The listing builds one solid part. Answer for the finished solid, in the listing's coordinates (mm). Face numbers are marked on the shaded views. A direction names the side the tool comes from. Give positions to 0.01 mm unless a question says otherwise; leave off trailing zeros. Write each loop counter-clockwise with the first axis right and the second up, starting at its lowest first coordinate (ties: lowest second). Pieces come first, ordered by that corner, then holes.
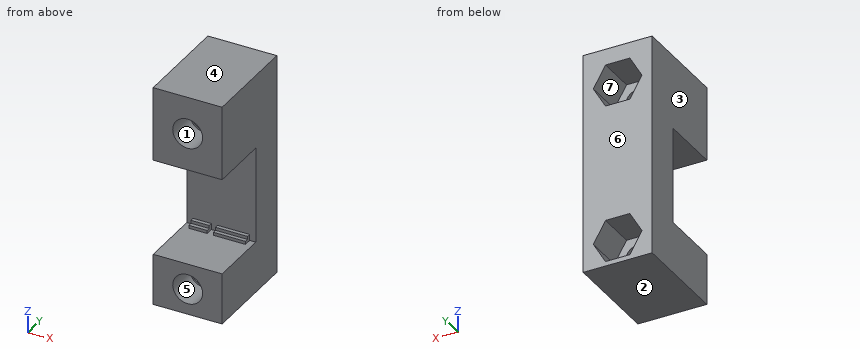
Autodesk Inventor part; units mm, degrees
ref_plane "YZ Plane" through (0, 0, 0) normal (1, 0, 0) x (0, 1, 0)
ref_plane "XZ Plane" through (0, 0, 0) normal (0, 1, 0) x (-1, 0, 0)
ref_plane "XY Plane" through (0, 0, 0) normal (0, 0, 1) x (1, 0, 0)
sketch "Szkic1" plane through (0, 0, 0) normal (1, 0, 0) x (0, 1, 0)
  line L0 (-4, 6.3) -> (4, 6.3)
  line L1 (4, 6.3) -> (4, -6.3)
  line L2 (4, -6.3) -> (-4, -6.3)
  line L3 (-4, 6.3) -> (-4, 13)
  line L4 (-4, -6.3) -> (-4, -13)
  line L5 (-1, -13) -> (-1, -9.3)
  line L6 (-1, -9.3) -> (7, -9.3)
  line L7 (7, -9.3) -> (7, 9.3)
  line L8 (7, 9.3) -> (-1, 9.3)
  line L9 (-1, 9.3) -> (-1, 13)
  line L10 (-4, 13) -> (-1, 13)
  line L11 (-4, -13) -> (-1, -13)
  point P0 (0, 0)
  point P1 (0, 6.3)
  point P2 (4, 0)
  dimension "d0" = 8
  dimension "d1" = 12.6
  dimension "d2" = 6.7
  dimension "d3" = 6.7
  dimension "d4" = 3
extrude "Wyciągnięcie proste1" add sketch "Szkic1" along normal blind 9
sketch "Szkic2" plane through (0, 4, -6.3) normal (0, -1, 0) x (1, 0, 0)
  line L0 (0, 12.6) -> (0, 0)
  line L1 (0, 0) -> (9, 0)
  line L2 (9, 12.6) -> (9, 0)
  line L3 (0, 12.6) -> (9, 12.6)
  line L4 (8.2, 12.6) -> (8.2, 0)
  line L5 (4, 12.6) -> (4, 0)
  line L6 (3.2, 12.6) -> (3.2, 0)
  line L7 (0.8, 0) -> (0.8, 12.6)
  line L8 (0.8, 12.6) -> (3.2, 12.6)
  line L9 (3.2, 12.6) -> (3.2, 11.8)
  line L10 (3.2, 11.8) -> (0.8, 11.8)
  line L11 (0.8, 11.8) -> (0.8, 12.6)
  line L12 (0.8, 0) -> (3.2, 0)
  line L13 (3.2, 0) -> (3.2, 0.8)
  line L14 (3.2, 0.8) -> (0.8, 0.8)
  line L15 (0.8, 0.8) -> (0.8, 0)
  line L16 (4, 12.6) -> (8.2, 12.6)
  line L17 (8.2, 12.6) -> (8.2, 11.8)
  line L18 (8.2, 11.8) -> (4, 11.8)
  line L19 (4, 11.8) -> (4, 12.6)
  line L20 (4, 0) -> (8.2, 0)
  line L21 (8.2, 0) -> (8.2, 0.8)
  line L22 (8.2, 0.8) -> (4, 0.8)
  line L23 (4, 0.8) -> (4, 0)
  point P0 (0, 6.3)
  point P1 (4, 0.8)
  point P2 (0.8, 0.8)
  point P3 (0.8, 11.8)
  dimension "d7" = 0.8
  dimension "d8" = 4.2
  dimension "d9" = 0.8
  dimension "d10" = 2.4
  dimension "d11" = 0.8
  dimension "d12" = 0.8
  dimension "d13" = 0.8
  dimension "d14" = 0.8
extrude "Wyciągnięcie proste2" add sketch "Szkic2" along normal blind 0.5 contours L3 L6 L10 L7 | L7 L14 L6 L1 | L3 L4 L18 L5 | L5 L22 L4 L1
sketch "Szkic3" plane through (0, 3.5, -6.3) normal (0, -1, 0) x (1, 0, 0)
  line L0 (8.2, 11.8) -> (8.2, 12.6)
  line L1 (4, 12.6) -> (8.2, 12.6)
  line L2 (4, 12.6) -> (4, 11.8)
  line L3 (4, 11.8) -> (8.2, 11.8)
  line L4 (3.2, 11.8) -> (3.2, 12.6)
  line L5 (0.8, 12.6) -> (3.2, 12.6)
  line L6 (0.8, 12.6) -> (0.8, 11.8)
  line L7 (0.8, 11.8) -> (3.2, 11.8)
  line L8 (0.8, 0.8) -> (0.8, 0)
  line L9 (3.2, 0) -> (0.8, 0)
  line L10 (3.2, 0) -> (3.2, 0.8)
  line L11 (3.2, 0.8) -> (0.8, 0.8)
  line L12 (4, 0.8) -> (4, 0)
  line L13 (8.2, 0) -> (4, 0)
  line L14 (8.2, 0) -> (8.2, 0.8)
  line L15 (8.2, 0.8) -> (4, 0.8)
  line L16 (8.2, 12.6) -> (8.2, 11.8)
  line L17 (8.2, 12.2) -> (0.8, 12.2)
  line L18 (8.2, 0.4) -> (0.8, 0.4)
  point P0 (0, 6.3)
  point P1 (4, 0.4)
  point P2 (3.2, 0.4)
  point P3 (4, 12.2)
  point P4 (3.2, 12.2)
extrude "Wyciągnięcie proste3" add sketch "Szkic3" along normal blind 0.5 contours L17 L6 L5 L4 | L17 L2 L1 L0 | L18 L14 L13 L12 | L18 L10 L9 L8
sketch "Szkic4" plane through (9, 0, 0) normal (1, 0, 0) x (0, 0, -1)
  line L0 (-6.3, -4) -> (-6.3, 4)
  line L1 (-6.3, 4) -> (6.3, 4)
  line L2 (6.3, 4) -> (6.3, -4)
  line L3 (6.3, -4) -> (13, -4)
  line L4 (13, -4) -> (13, -1)
  line L5 (13, -1) -> (9.3, -1)
  line L6 (9.3, -1) -> (9.3, 7)
  line L7 (9.3, 7) -> (-9.3, 7)
  line L8 (-9.3, 7) -> (-9.3, -1)
  line L9 (-9.3, -1) -> (-13, -1)
  line L10 (-13, -1) -> (-13, -4)
  line L11 (-13, -4) -> (-6.3, -4)
  line L12 (-13, -1) -> (13, -1)
  line L13 (13, -1) -> (13, 9)
  line L14 (13, 9) -> (-13, 9)
  line L15 (-13, 9) -> (-13, -1)
  point P0 (0, 0)
  dimension "d19" = 10
extrude "Wyciągnięcie proste4" add sketch "Szkic4" against normal up to surface (9 mm away) contours L9 L15 L14 L13 L5 L6 L7 L8
sketch "Szkic5" plane through (0, -4, 13) normal (0, 0, 1) x (1, 0, 0)
  line L0 (0, 0) -> (0, 13)
  line L1 (0, 0) -> (9, 0)
  line L2 (9, 13) -> (9, 0)
  line L3 (9, 13) -> (0, 13)
  point P0 (0, 4)
extrude "Wyciągnięcie proste5" add sketch "Szkic5" along normal blind 3
sketch "Szkic6" plane through (0, -4, -13) normal (0, -1, 0) x (1, 0, 0)
  line L0 (0, 0) -> (9, 0)
  line L1 (0, 6.7) -> (9, 6.7)
  line L2 (0, 19.3) -> (9, 19.3)
  line L3 (0, 29) -> (9, 29)
  line L4 (4.5, 0) -> (4.5, 6.7) construction
  line L5 (4.5, 19.3) -> (4.5, 29) construction
  point P0 (0, 13)
  point P1 (4.5, 3.35)
  point P2 (4.5, 24.15)
hole "Otwór1" at (4.5, -4, -9.65) at (4.5, -4, 11.15) direction (0, 1, 0) diameter 3.5 depth 8 counterbore diameter 3.9 counterbore depth 4
sketch "Szkic7" plane through (0, 9, -13) normal (0, 1, 0) x (1, 0, 0)
  circle A0 centre (4.5, -3.35) radius 1.75
  circle A1 centre (4.5, -24.15) radius 1.75
  circle A2 centre (4.5, -3.35) radius 2.75
  circle A3 centre (4.5, -24.15) radius 2.75
  line L0 (6.0877, -0.6) -> (7.6754, -3.35)
  line L1 (7.6754, -3.35) -> (6.0877, -6.1)
  line L2 (6.0877, -6.1) -> (2.9123, -6.1)
  line L3 (2.9123, -6.1) -> (1.3246, -3.35)
  line L4 (1.3246, -3.35) -> (2.9123, -0.6)
  line L5 (2.9123, -0.6) -> (6.0877, -0.6)
  line L6 (2.9123, -26.9) -> (1.3246, -24.15)
  line L7 (1.3246, -24.15) -> (2.9123, -21.4)
  line L8 (2.9123, -21.4) -> (6.0877, -21.4)
  line L9 (6.0877, -21.4) -> (7.6754, -24.15)
  line L10 (7.6754, -24.15) -> (6.0877, -26.9)
  line L11 (6.0877, -26.9) -> (2.9123, -26.9)
  point P0 (0, -13)
  point P1 (4.5, -0.6)
  point P2 (4.5, -26.9)
  dimension "d31" = 5.5
  dimension "d32" = 5.5
extrude "Wyciągnięcie proste6" cut sketch "Szkic7" against normal blind 5 contours A0 | A1 | A2 | A2 L0 L1 | A2 L5 L0 | L1 L2 A2 | A2 L4 L5 | L2 L3 A2 | A2 L3 L4 | A3 | A3 L9 L10 | A3 L8 L9 | L10 L11 A3 | A3 L7 L8 | L11 L6 A3 | A3 L6 L7
properties part number "motor_bracket"
Item 1: A cutting plane is placed at B-B, the plane y = 5. Give the vertices of the cut face in (x, z).
Conclusion:
outline: (0, -13) - (9, -13) - (9, 16) - (0, 16) - close; hole (1.32, -9.65) - (2.91, -12.4) - (6.09, -12.4) - (7.68, -9.65) - (6.09, -6.9) - (2.91, -6.9) - close; hole (1.32, 11.15) - (2.91, 8.4) - (6.09, 8.4) - (7.68, 11.15) - (6.09, 13.9) - (2.91, 13.9) - close
Item 2: Consider probe 1 along Z at (x, y) = (3.75, 4.75); probe 2 along Z at (x, y) = (4.5, -1.8); probe 3 along Z at (x, y) = (4.5, 2.1). Determine where each line is inside the solid, lowest interval first.
Conclusion:
probe 1: z = -13 to -12.4, -6.9 to 8.4, 13.9 to 16
probe 2: z = -13 to -11.6, -7.7 to -6.3, 6.3 to 9.2, 13.1 to 16
probe 3: z = -13 to -11.4, -7.9 to -6.3, 6.3 to 9.4, 12.9 to 16
Item 3: Determine the mould class of the marked faces 1, 2, 3 and 4 for opening direction Z: pulls with the +Z half, pulls with the -Z half, needs draft (parallel to the pull), parting line crosses it, or undercut.
Conclusion:
face 1: undercut
face 2: pulls with the -Z half
face 3: needs draft
face 4: pulls with the +Z half
Item 4: Which of the six approach directions +Z, -Z, +X, -X, +Y, -Y give full straight-line access (tool end or side, diameter ignored) to the marked faces 5, 6 and 7?
Conclusion:
face 5: -Y
face 6: +Z, -Z, +X, -X, +Y
face 7: +Y
Item 5: A cutting plane is placed at A-A, the plane y = -1.5. Give the vertices of the cut face in (x, z), plus the area to 3 significant figures.
Conclusion:
outline: (0, -13) - (9, -13) - (9, -6.3) - (0, -6.3) - close; (0, 6.3) - (9, 6.3) - (9, 16) - (0, 16) - close; hole circle Ø3.9 at (4.5, -9.65); hole circle Ø3.9 at (4.5, 11.15)
area: 124 mm2
Item 6: A cutting plane is placed at C-C, the plane z = -11. Give the vertices of the cut face in (x, y).
Conclusion:
outline: (0, -4) - (3.09, -4) - (3.09, 0) - (3.39, 0) - (3.39, 4) - (2.1, 4) - (2.1, 9) - (0, 9) - close; (5.61, 0) - (5.91, 0) - (5.91, -4) - (9, -4) - (9, 9) - (6.9, 9) - (6.9, 4) - (5.61, 4) - close
Item 7: Each of these flat-tipped pins is pushed along its axis until it touches: P1, Ø2, axis at x = 2, z = -3, coming from the -Y side; P2, Ø2, axis at x = 5.5, z = -5, coming from the -Y side. Where does it stop, or does it pass through?
Conclusion:
P1: stops at y = 4
P2: stops at y = 3
Item 8: A cutting plane is placed at D-D, the plane x = 0.5. Give the vertices of the cut face in (y, z), plus the area to 3 significant figures.
Conclusion:
outline: (-4, -13) - (9, -13) - (9, 16) - (-4, 16) - (-4, 6.3) - (4, 6.3) - (4, -6.3) - (-4, -6.3) - close
area: 276 mm2
